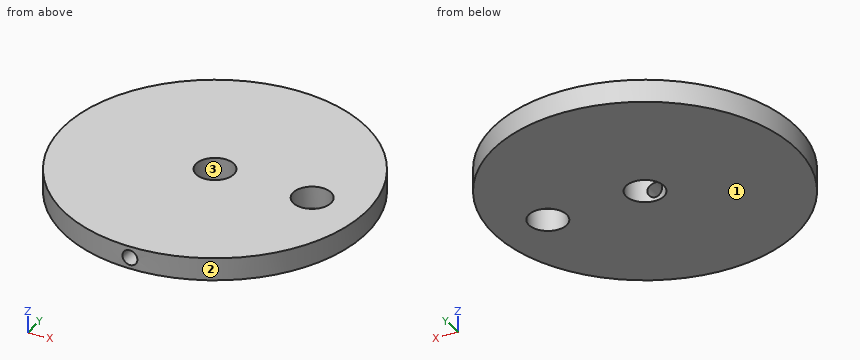
from build123d import *

# Parameters (mm, degrees)
SKETCH_1_R          = 20
EXTRUDE_1_DEPTH     = 3
SKETCH_2_R          = 2.5
CUT_EXTRUDE_1_DEPTH = 29.442925307
SKETCH_4_R          = 2.5
CUT_EXTRUDE_2_DEPTH = 29.442925307
F_2_0MM_1_REACH     = 46.747
F_2_0MM_1_BORE_R    = 1


with BuildPart() as part:
    # 草图1 → 凸台-拉伸1 (new body)
    with BuildSketch(Plane.XY):
        Circle(SKETCH_1_R)
    extrude(amount=EXTRUDE_1_DEPTH)

    # 草图2 → 切除-拉伸1 (cut, through all)
    with BuildSketch(Plane.XY.offset(3)):
        Circle(SKETCH_2_R)
    extrude(amount=-CUT_EXTRUDE_1_DEPTH, mode=Mode.SUBTRACT)

    # 草图4 → 切除-拉伸2 (cut, through all)
    with BuildSketch(Plane.XY.offset(3)):
        with Locations((13, 0)):
            Circle(SKETCH_4_R)
    extrude(amount=-CUT_EXTRUDE_2_DEPTH, mode=Mode.SUBTRACT)

    # Ø2.0mm 暗销孔1 bore (on position points) → Ø2.0mm 暗销孔1 (cut, up to next)
    with BuildSketch(Plane(origin=(0, -20, 1.5), x_dir=(-1, 0, 0), z_dir=(0, -1, 0)), mode=Mode.PRIVATE) as f_2_0mm_1_sk1:
        Circle(F_2_0MM_1_BORE_R)
    f_2_0mm_1_tool1 = extrude(f_2_0mm_1_sk1.sketch, amount=-F_2_0MM_1_REACH, mode=Mode.PRIVATE) & part.part
    add(f_2_0mm_1_tool1.solids().sort_by_distance((0, -20, 1.5))[0], mode=Mode.SUBTRACT)


solid = part.part
The model under review builds one solid part; all positions refer to its coordinate system, in mm. Face numbers are marked on the shaded views. Round coordinates to 2 decimals unless told otherwise and drop trailing zeros. Write each loop counter-clockwise with the first axis right and the second up, starting at its lowest first coordinate (ties: lowest second). Pieces come first, ordered by that corner, then holes. Notation, with made-up numbers: (-23, 47) -> (-6, 47) arc R13 ccw to (-6, 67) -> close; hole circle Ø6 at (49, 4). An arc over 180 degrees is marked (long way). Answer as a JSON object with one key per item and string values.
1. The part is to be moulded in two halves that separate along Y. For the marked faces 1, 2 and 3, say which applies: pulls with the +Y half, pulls with the -Y half, needs draft (parallel to the pull), parting line crosses it, or undercut.
Results found:
{"face 1": "needs draft", "face 2": "parting line crosses it", "face 3": "undercut"}
2. We need section B-B on x = 0. State the section outline as (y, z) points, and give its area (3 significant figures).
Results found:
{"outline": "(-20, 0) -> (-2.5, 0) -> (-2.5, 0.5) -> (-20, 0.5) -> close; (-20, 2.5) -> (-2.5, 2.5) -> (-2.5, 3) -> (-20, 3) -> close; (2.5, 0) -> (20, 0) -> (20, 3) -> (2.5, 3) -> close", "area": "70.0 mm^2"}
3. We need section D-D on y = -14.5. State the section outline as (x, z) points.
Results found:
{"outline": "(-13.77, 0) -> (13.77, 0) -> (13.77, 3) -> (-13.77, 3) -> close; hole circle Ø2 at (0, 1.5)"}
4. Clearance check with a flat-ended pin moving along its axis: pin 1 (4.5 mm diameter, centred on x = 0, y = 0, fed in from -Z). State where the tip first meets the part, or that it passes through.
Results found:
{"pin 1": "passes through"}
5. We need section C-C on x = 13. State the section outline as (y, z) points.
Results found:
{"outline": "(-15.2, 0) -> (-2.5, 0) -> (-2.5, 3) -> (-15.2, 3) -> close; (2.5, 0) -> (15.2, 0) -> (15.2, 3) -> (2.5, 3) -> close"}
6. To check wall thickness, follow line 1 along Z through (x, y) = (0, -14.5); line 2 along Y through (x, z) = (13, 1.85); line 3 along Y through (x, z) = (0, 2). State the ranges of each line that lie inside material, in increasing order.
Results found:
{"line 1": "z = 0 to 0.5, 2.5 to 3", "line 2": "y = -15.2 to -2.5, 2.5 to 15.2", "line 3": "y = 2.5 to 20"}
7. We need section A-A on y = 0. State the section outline as (x, z) points, and give its area (3 significant figures).
Results found:
{"outline": "(-20, 0) -> (-2.5, 0) -> (-2.5, 3) -> (-20, 3) -> close; (2.5, 0) -> (10.5, 0) -> (10.5, 3) -> (2.5, 3) -> close; (15.5, 0) -> (20, 0) -> (20, 3) -> (15.5, 3) -> close", "area": "90.0 mm^2"}
